Check sheet for the modelled part. Datum: model origin and axes. Units: mm. Coordinates: 2 decimals unless noted, no trailing zeros. Loops run counter-clockwise (first coordinate to the right, second up) from the corner with the lowest first, then second, coordinate; pieces in that order, holes last. Notation, with made-up numbers: (63.5, 16.25) -> (76.5, 16.25) arc R9 cw to (76.5, 33.25) -> close; hole circle Ø2 at (68, 22.5). An arc over 180 degrees is marked (long way). Use one line per item in the form item = value.
Autodesk Inventor part; units mm, degrees
ref_plane "YZ Plane" through (0, 0, 0) normal (1, 0, 0) x (0, 1, 0)
ref_plane "XZ Plane" through (0, 0, 0) normal (0, 1, 0) x (-1, 0, 0)
ref_plane "XY Plane" through (0, 0, 0) normal (0, 0, 1) x (1, 0, 0)
sketch "Sketch1" plane through (0, 0, 0) normal (1, 0, 0) x (0, 1, 0)
  line L0 (0, 0) -> (-127, 0)
  line L1 (-127, 0) -> (-127, 127)
  line L2 (-127, 127) -> (0, 127)
  line L3 (0, 127) -> (0, 0)
  line L4 (-19.05, 65.151) -> (-120.65, 65.151)
  line L5 (-120.65, 65.151) -> (-120.65, 61.849)
  line L6 (-120.65, 61.849) -> (-19.05, 61.849)
  line L7 (-19.05, 61.849) -> (-19.05, 65.151)
  line L8 (0, 47.625) -> (-12.7, 47.625)
  line L9 (-12.7, 47.625) -> (-12.7, 79.375)
  line L10 (-12.7, 79.375) -> (0, 79.375)
  line L11 (0, 79.375) -> (0, 47.625)
  line L12 (-12.7, 47.625) -> (-12.7, 0)
  line L13 (-12.7, 79.375) -> (-12.7, 127)
  dimension "d0" = 127
  dimension "d1" = 127
  dimension "d2" = 6.35
  dimension "d4" = 3.302
  dimension "d5" = 61.849
  dimension "d25" = 12.7
  dimension "d26" = 31.75
  dimension "d27" = 47.625
  dimension "d28" = 6.35
extrude "Extrusion1" add sketch "Sketch1" along normal blind 3.175 contours L0 L1 L2 L13 L9 L12
sketch "Sketch3" plane through (0, 0, 0) normal (-1, 0, 0) x (0, 0, 1)
  circle A0 centre (34.925, -41.275) radius 2.5797
  line L0 (0, -127) -> (0, -12.7)
  line L1 (0, -12.7) -> (0, 0)
  line L2 (0, 0) -> (20.4302, 0)
  line L3 (20.4302, 0) -> (0, -12.7)
  circle A1 centre (34.925, -98.425) radius 2.5797
  circle A2 centre (92.075, -41.275) radius 2.5797
  circle A3 centre (92.075, -98.425) radius 2.5797
  line L4 (0, -12.7) -> (127, -12.7)
  dimension "d31" = 57.15
  dimension "d34" = 57.15
  dimension "d37" = 34.925
  dimension "d38" = 28.575
  dimension "d39" = 5.1594
extrude "Extrusion4" cut sketch "Sketch3" against normal through all contours A0 | A1 | A2 | A3
fillet "Fillet5" radius 3.175 1 edges at (3.175, -12.7, 63.5)
equation "\"d5\" = -0.5 * d4 + 0.5 * d1"
equation "\"d27\" = -0.5 * d26 + 0.5 * d1"
equation "\"d28\" = d2"
properties part number "Gripper plate"
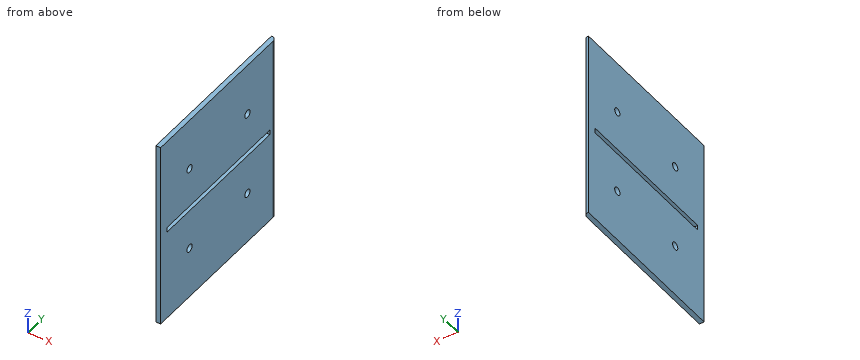
(1) Scan lines: line 1 along Z through (x, y) = (1.45, -77); line 2 along Y through (x, z) = (0.4, 90); line 3 along Z through (x, y) = (1.3, -97.5). Record each from-to range of solid material in increasing order.
Established:
line_1 = 0 to 61.85, 65.15 to 127
line_2 = -127 to -99.96, -96.89 to -42.81, -39.74 to -12.73
line_3 = 0 to 32.52, 37.33 to 61.85, 65.15 to 89.67, 94.48 to 127
(2) Section check A-A, the plane y = -61.5. Record the boundary of the cut face in (x, z) (3 decimals).
Established:
outline = (0, 0) -> (3.175, 0) -> (3.175, 61.849) -> (0, 61.849) -> close; (0, 65.151) -> (3.175, 65.151) -> (3.175, 127) -> (0, 127) -> close
(3) Section check C-C, the plane z = 35.5. Give the number of separate pieces and of enclosed holes in the cut face, plus the area to 3 significant figures.
Established:
separate_pieces = 3
enclosed_holes = 0
area = 329 mm²
(4) Section check B-B, the plane x = 1.45. Record the boundary of the cut face in (y, z) (3 decimals), plus the area to 3 significant figures.
Established:
outline = (-127, 0) -> (-13.05, 0) -> (-13.05, 127) -> (-127, 127) -> close; hole (-120.65, 61.849) -> (-19.05, 61.849) -> (-19.05, 65.151) -> (-120.65, 65.151) -> close; hole circle Ø5.159 at (-98.425, 34.925); hole circle Ø5.159 at (-98.425, 92.075); hole circle Ø5.159 at (-41.275, 34.925); hole circle Ø5.159 at (-41.275, 92.075)
area = 14,100 mm²
(5) Go/stop test with flat-tipped pins: P1, Ø1.5, axis at y = -109.5, z = 113.5, coming from the -X side; P2, Ø4, axis at y = -98.425, z = 92.075, coming from the -X side; P3, Ø1.6, axis at x = 2, z = 64, coming from the +Y side. Record where each tip stops, or that it passes through.
Established:
P1 = 0
P2 = through
P3 = -12.94
